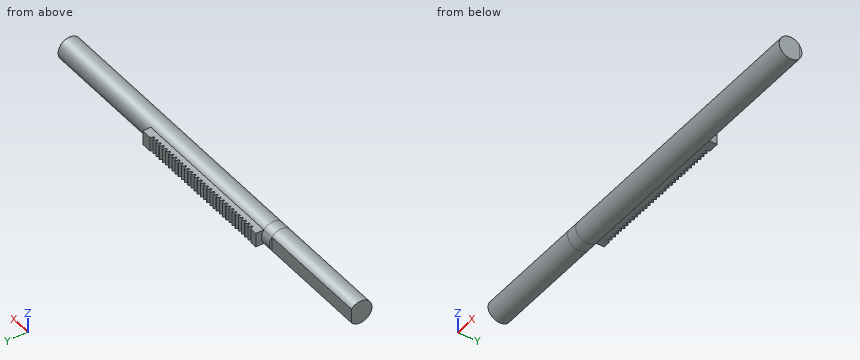
```python
from build123d import *
from build123d.topology import SkipClean

# Parameters (mm, degrees)
SKETCH1_W                = 150
SKETCH1_H                = 7
BOSS_EXTRUDE2_DEPTH      = 6.25
CUT_EXTRUDE1_DEPTH       = 140.036501376
LPATTERN1_COUNT          = 32
LPATTERN1_PITCH          = 3.92
CUT_EXTRUDE2_START       = -6.25
CUT_EXTRUDE2_OUTLINE_W   = 4.009572156
CUT_EXTRUDE2_OUTLINE_H   = 7
CUT_EXTRUDE2_OUTLINE_W_2 = 6
CUT_EXTRUDE2_DEPTH       = 12.5
BOSS_EXTRUDE3_DEPTH      = 112
BOSS_EXTRUDE3_DEPTH_BACK = 248.5
SKETCH7_R                = 10
BOSS_EXTRUDE4_DEPTH      = 111.735590033
SKETCH8_R                = 6
CUT_EXTRUDE3_DEPTH       = 22
BOSS_EXTRUDE5_START      = 10
SKETCH10_R               = 10
BOSS_EXTRUDE5_DEPTH      = 10
CUT_EXTRUDE5_START       = -22
SKETCH11_R               = 6
CUT_EXTRUDE5_DEPTH       = 22


# Read off the part's stored shape, not the designer's step: Cut-Extrude2
with BuildPart() as part:
    # Sketch1 → Boss-Extrude2 (new, symmetric)
    with BuildSketch(Plane.XY):
        with Locations((63.159569831, 10.783538746)):
            Rectangle(SKETCH1_W, SKETCH1_H)
    extrude(amount=BOSS_EXTRUDE2_DEPTH, both=True)

    # Sketch2 → Cut-Extrude1 (cut, symmetric)
    with BuildSketch(Plane.XY):
        with BuildLine():
            ThreePointArc((0.615260942, 11.545117419), (0, 11.5615), (-0.615260942, 11.545117419))
            ThreePointArc((-0.615260942, 11.545117419), (-1.023565158, 13.002884474), (-1.830858013, 14.283538746))
            ThreePointArc((-1.830858013, 14.283538746), (0, 14.4004), (1.830858013, 14.283538746))
            ThreePointArc((1.830858013, 14.283538746), (1.023565158, 13.002884474), (0.615260942, 11.545117419))
        make_face()
    cut_extrude1 = extrude(amount=CUT_EXTRUDE1_DEPTH, both=True, mode=Mode.SUBTRACT)

    # LPattern1: Cut-Extrude1 ×32
    with Locations(*[(i * LPATTERN1_PITCH, 0, 0) for i in range(1, LPATTERN1_COUNT)]):
        add(cut_extrude1, mode=Mode.SUBTRACT)

    # Cut-Extrude2 outline → Cut-Extrude2 (cut)
    with BuildSketch(Plane.XY.offset(CUT_EXTRUDE2_START)):
        with Locations((-9.835644091, 10.783538746)):
            Rectangle(CUT_EXTRUDE2_OUTLINE_W, CUT_EXTRUDE2_OUTLINE_H)
        with Locations((135.159569831, 10.783538746)):
            Rectangle(CUT_EXTRUDE2_OUTLINE_W_2, CUT_EXTRUDE2_OUTLINE_H)
    extrude(amount=CUT_EXTRUDE2_DEPTH, mode=Mode.SUBTRACT)

    # Sketch5 → Boss-Extrude3 (add, two sides: drawn at the far end of the back side and taken through both)
    with BuildSketch(Plane(origin=(132.159569831, 0, 0), x_dir=(0, 0, -1), z_dir=(1, 0, 0)).offset(-BOSS_EXTRUDE3_DEPTH_BACK)):
        with BuildLine():
            Line((6.25, 7.283538746), (-6.25, 7.283538746))
            ThreePointArc((-6.25, 7.283538746), (0, -10.522708752), (6.25, 7.283538746))
        make_face()
    extrude(amount=BOSS_EXTRUDE3_DEPTH + BOSS_EXTRUDE3_DEPTH_BACK)

    # Sketch7 → Boss-Extrude4 (add)
    with BuildSketch(Plane(origin=(132.159569831, 0, 0), x_dir=(0, 0, -1), z_dir=(1, 0, 0))):
        with Locations(Location((0, -0.522708752, 0), (0, 0, 128.682187453))):
            Circle(SKETCH7_R)
    extrude(amount=BOSS_EXTRUDE4_DEPTH)

    # Sketch8 → Cut-Extrude3 (cut)
    with BuildSketch(Plane(origin=(243.895159863, 0, 0), x_dir=(0, 0, -1), z_dir=(1, 0, 0))):
        with Locations(Location((0, -0.522708752, 0), (0, 0, 90))):
            Circle(SKETCH8_R)
    extrude(amount=-CUT_EXTRUDE3_DEPTH, mode=Mode.SUBTRACT)

    # Sketch10 → Boss-Extrude5 (add)
    with SkipClean():  # the faces are left unmerged after this step: merging them gives an invalid solid
        with BuildSketch(Plane.ZY.offset(7.830858013).offset(BOSS_EXTRUDE5_START)):
            with Locations(Location((0, -0.522708752, 0), (0, 0, 128.682187453))):
                Circle(SKETCH10_R)
        extrude(amount=-BOSS_EXTRUDE5_DEPTH)
    add(part.part.scale(1), mode=Mode.REPLACE)  # the faces are merged on a copy

    # Sketch11 → Cut-Extrude5 (cut)
    with BuildSketch(Plane.ZY.offset(17.830858013).offset(CUT_EXTRUDE5_START)):
        with Locations(Location((0, -0.522708752, 0), (0, 0, 90))):
            Circle(SKETCH11_R)
    extrude(amount=CUT_EXTRUDE5_DEPTH, mode=Mode.SUBTRACT)


solid = part.part
```
For this review, take the finished solid that the model builds, in its own axes (mm). Round coordinates to 2 decimals unless told otherwise and drop trailing zeros. Write each loop counter-clockwise with the first axis right and the second up, starting at its lowest first coordinate (ties: lowest second). Pieces come first, ordered by that corner, then holes. Notation, with made-up numbers: (65.5, -1) - (93.5, -1) arc R13 cw to (93.5, 18) - close; hole circle Ø4 at (67.5, 12). An arc over 180 degrees is marked (long way). Answer as CSV lines item,"result". Start each with the question number.
(1) Add section D-D, the plane x = 215.5. State the section outline as (y, z) points.
(2) Add section A-A, the plane y = 2. State the section outline as (x, z) points, plus the area to 3 significant figures.
(3) Add section C-C, the plane x = -26.5. State the section outline as (y, z) points.
(4) For pin 1 (1.1 mm diameter, centred on y = 8, z = 2, fed in from -X); pin 2 (5 mm diameter, centred on y = 8, z = 1, fed in from +X); pin 3 (0.7 mm diameter, centred on y = 8, z = -2.5, fed in from +X); pin 4 (3.5 mm diameter, centred on x = 74.5, y = 10, fed in from +Z), all flat-tipped, find the tip position at first contact; note any pin that passes through.
(5) For line 1 (X direction, y = 1.25, z = -1.5); line 2 (Z direction, x = 80, y = 7.75); line 3 (Z direction, x = 197, y = -1.25), list the stretches that pass through material, from the lowest coordinate up.
(6) Add section B-B, the plane z = 0. State how many separate pieces and enclosed holes the cut face has, plus the area to 3 significant figures.
From the geometry:
1,outline,"circle Ø20 at (-0.52, 0)"
2,outline,"(-116.34, -9.68) - (244.16, -9.68) - (244.16, 9.68) - (-116.34, 9.68) - close; hole (-17.83, -5.44) - (4.17, -5.44) - (4.17, 5.44) - (-17.83, 5.44) - close; hole (221.9, -5.44) - (243.9, -5.44) - (243.9, 5.44) - (221.9, 5.44) - close"
2,area,"6,500 mm²"
3,outline,"(7.28, -6.25) - (7.28, 6.25) arc R10 ccw (long way) to start"
4,pin 1,"stops at x = -17.83"
4,pin 2,"stops at x = 244.16"
4,pin 3,"stops at x = 243.9"
4,pin 4,"stops at z = 6.25"
5,line 1,"x = -116.34 to -17.83, 4.17 to 221.9, 243.9 to 244.16"
5,line 2,"z = -6.25 to 6.25"
5,line 3,"z = -9.97 to 9.97"
6,separate pieces,"1"
6,enclosed holes,"2"
6,area,"6,950 mm²"
